```python
from build123d import *

# Parameters (mm, degrees)
SKETCH1_W           = 37.9349
SKETCH1_H           = 37.9349
BOSS_EXTRUDE1_DEPTH = 3.175
SKETCH9_R           = 1.1176
CUT_EXTRUDE2_DEPTH  = 3.175
SKETCH10_R          = 7.493
CUT_EXTRUDE3_DEPTH  = 3.175
SKETCH11_W          = 10.4648
SKETCH11_H          = 1.8796
BOSS_EXTRUDE2_DEPTH = 3.175


with BuildPart() as part:
    # Sketch1 → Boss-Extrude1 (new body)
    with BuildSketch(Plane.XY):
        with Locations((18.96745, 18.96745)):
            Rectangle(SKETCH1_W, SKETCH1_H)
    extrude(amount=BOSS_EXTRUDE1_DEPTH)

    # Sketch9 → Cut-Extrude2 (cut)
    with BuildSketch(Plane.XY.offset(3.175)):
        with Locations((33.62325, 33.62325)):
            Circle(SKETCH9_R)
        with Locations((4.31165, 33.62325)):
            Circle(SKETCH9_R)
        with Locations((4.31165, 4.31165)):
            Circle(SKETCH9_R)
        with Locations((33.62325, 4.31165)):
            Circle(SKETCH9_R)
        with BuildLine():
            Line((35.385619933, 12.100169933), (35.385619933, 2.549280067))
            Line((35.385619933, 2.549280067), (25.834730067, 2.549280067))
            ThreePointArc((25.834730067, 2.549280067), (25.2984, 2.01295), (25.834730067, 1.476619933))
            Line((25.834730067, 1.476619933), (35.385619933, 1.476619933))
            ThreePointArc((35.385619933, 1.476619933), (37.303202335, 0.631697665), (36.458280067, 2.549280067))
            Line((36.458280067, 2.549280067), (36.458280067, 12.100169933))
            ThreePointArc((36.458280067, 12.100169933), (35.92195, 12.6365), (35.385619933, 12.100169933))
        make_face()
        with BuildLine():
            Line((35.385619933, 36.458280067), (25.834730067, 36.458280067))
            ThreePointArc((25.834730067, 36.458280067), (25.2984, 35.92195), (25.834730067, 35.385619933))
            Line((25.834730067, 35.385619933), (35.385619933, 35.385619933))
            Line((35.385619933, 35.385619933), (35.385619933, 25.834730067))
            ThreePointArc((35.385619933, 25.834730067), (35.92195, 25.2984), (36.458280067, 25.834730067))
            Line((36.458280067, 25.834730067), (36.458280067, 35.385619933))
            ThreePointArc((36.458280067, 35.385619933), (37.303202335, 37.303202335), (35.385619933, 36.458280067))
        make_face()
        with BuildLine():
            Line((12.048880067, 36.458280067), (2.549280067, 36.458280067))
            ThreePointArc((2.549280067, 36.458280067), (0.631697665, 37.303202335), (1.476619933, 35.385619933))
            Line((1.476619933, 35.385619933), (1.476619933, 25.886019933))
            ThreePointArc((1.476619933, 25.886019933), (2.01295, 25.349689867), (2.549280067, 25.886019933))
            Line((2.549280067, 25.886019933), (2.549280067, 35.385619933))
            Line((2.549280067, 35.385619933), (12.048880067, 35.385619933))
            ThreePointArc((12.048880067, 35.385619933), (12.585210133, 35.92195), (12.048880067, 36.458280067))
        make_face()
        with BuildLine():
            Line((23.06955, 36.458280067), (14.86535, 36.458280067))
            ThreePointArc((14.86535, 36.458280067), (14.329019933, 35.92195), (14.86535, 35.385619933))
            Line((14.86535, 35.385619933), (23.06955, 35.385619933))
            ThreePointArc((23.06955, 35.385619933), (23.605880067, 35.92195), (23.06955, 36.458280067))
        make_face()
        with BuildLine():
            Line((2.549280067, 23.06955), (2.549280067, 14.86535))
            ThreePointArc((2.549280067, 14.86535), (2.01295, 14.329019933), (1.476619933, 14.86535))
            Line((1.476619933, 14.86535), (1.476619933, 23.06955))
            ThreePointArc((1.476619933, 23.06955), (2.01295, 23.605880067), (2.549280067, 23.06955))
        make_face()
        with BuildLine():
            Line((36.458280067, 23.06955), (36.458280067, 14.86535))
            ThreePointArc((36.458280067, 14.86535), (35.92195, 14.329019933), (35.385619933, 14.86535))
            Line((35.385619933, 14.86535), (35.385619933, 23.06955))
            ThreePointArc((35.385619933, 23.06955), (35.92195, 23.605880067), (36.458280067, 23.06955))
        make_face()
        with BuildLine():
            Line((23.06955, 2.549280067), (14.86535, 2.549280067))
            ThreePointArc((14.86535, 2.549280067), (14.329019933, 2.01295), (14.86535, 1.476619933))
            Line((14.86535, 1.476619933), (23.06955, 1.476619933))
            ThreePointArc((23.06955, 1.476619933), (23.605880067, 2.01295), (23.06955, 2.549280067))
        make_face()
        with BuildLine():
            Line((2.549280067, 12.100169933), (2.549280067, 2.549280067))
            Line((2.549280067, 2.549280067), (12.100169933, 2.549280067))
            ThreePointArc((12.100169933, 2.549280067), (12.6365, 2.01295), (12.100169933, 1.476619933))
            Line((12.100169933, 1.476619933), (2.600569933, 1.476619933))
            ThreePointArc((2.600569933, 1.476619933), (0.681867267, 0.681867267), (1.476619933, 2.600569933))
            Line((1.476619933, 2.600569933), (1.476619933, 12.100169933))
            ThreePointArc((1.476619933, 12.100169933), (2.01295, 12.6365), (2.549280067, 12.100169933))
        make_face()
    extrude(amount=-CUT_EXTRUDE2_DEPTH, mode=Mode.SUBTRACT)

    # Sketch10 → Cut-Extrude3 (cut)
    with BuildSketch(Plane(origin=(0, 0, 0), x_dir=(-1, 0, 0), z_dir=(0, 0, -1))):
        with Locations((-18.96745, 18.96745)):
            Circle(SKETCH10_R)
    extrude(amount=-CUT_EXTRUDE3_DEPTH, mode=Mode.SUBTRACT)

    # Sketch11 → Boss-Extrude2 (add)
    with BuildSketch(Plane.XY.offset(3.175)):
        with Locations((-5.2324, 25.8191)):
            Rectangle(SKETCH11_W, SKETCH11_H)
        with Locations((-5.2324, 12.1158)):
            Rectangle(SKETCH11_W, SKETCH11_H)
    extrude(amount=-BOSS_EXTRUDE2_DEPTH)


solid = part.part
```
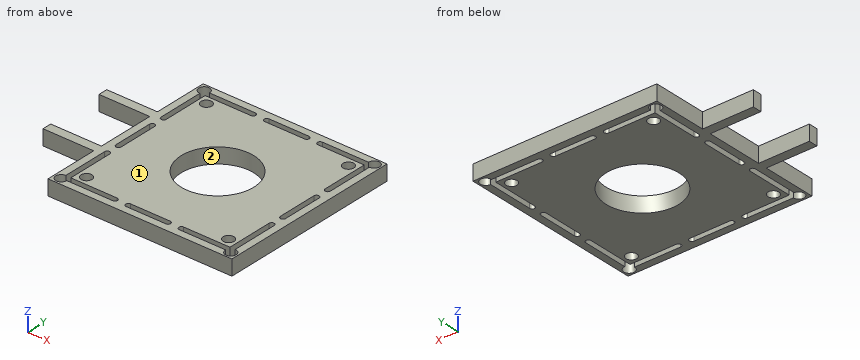
Could you check a few things on this model? Use its own coordinates, in mm. Face numbers are marked on the shaded views. Round coordinates to 2 decimals unless told otherwise and drop trailing zeros. Loops run counter-clockwise (first coordinate to the right, second up) from the corner with the lowest first, then second, coordinate; pieces in that order, holes last. Notation, with made-up numbers: M 80.25,-30 L 115.25,-30 A25 ccw 115.25,2 Z; hole C -10.75,11.5 d10. An arc over 180 degrees is marked long. Put each result on its own line as item: value.
Q1. Imagine slicing it at D-D (x = 22.5). Write out the boundary of the cut face in (y, z) (3 decimals).
Check result:
outline: M 0,0 L 1.477,0 L 1.477,3.175 L 0,3.175 Z; M 2.549,0 L 12.359,0 L 12.359,3.175 L 2.549,3.175 Z; M 25.575,0 L 35.386,0 L 35.386,3.175 L 25.575,3.175 Z; M 36.458,0 L 37.935,0 L 37.935,3.175 L 36.458,3.175 Z
Q2. Thinking about a two-plate mould opening in Y: for the marked faces 1 and 2, which applies, released by +Y, released by -Y, zero draft, split by the parting line, or undercut?
Check result:
face 1: zero draft
face 2: undercut
Q3. I need wall thicknesses on probe 1 along X at (y, z) = (35, 0.9); probe 2 along X at (y, z) = (19, 0.6). Which ranges of each line are inside material? Lowest first, please.
Check result:
probe 1: 0 to 1.48, 2.55 to 35.39, 36.46 to 37.93
probe 2: 0 to 1.48, 2.55 to 11.47, 26.46 to 35.39, 36.46 to 37.93
Q4. For pin 1 (1 mm diameter, centred on y = 7.5, z = 2, fed in from -X); pin 2 (2 mm diameter, centred on x = 36.51, y = 1.43, fed in from -Z); pin 3 (1 mm diameter, centred on x = -4, z = 1, fed in from -Y), each with a flat end and sliding along its axis, tell me the tip position at first contact or that it passes through.
Check result:
pin 1: x = 0
pin 2: through
pin 3: y = 11.18
Q5. Imagine slicing it at C-C (y = 16). Write out the boundary of the cut face in (x, z) (3 decimals), then the cut area to 3 significant figures.
Check result:
outline: M 0,0 L 1.477,0 L 1.477,3.175 L 0,3.175 Z; M 2.549,0 L 12.087,0 L 12.087,3.175 L 2.549,3.175 Z; M 25.848,0 L 35.386,0 L 35.386,3.175 L 25.848,3.175 Z; M 36.458,0 L 37.935,0 L 37.935,3.175 L 36.458,3.175 Z
area: 69.9 mm2
Q6. Imagine slicing it at A-A (x = 27.5). Write out the boundary of the cut face in (y, z) (3 decimals).
Check result:
outline: M 0,0 L 1.477,0 L 1.477,3.175 L 0,3.175 Z; M 2.549,0 L 35.386,0 L 35.386,3.175 L 2.549,3.175 Z; M 36.458,0 L 37.935,0 L 37.935,3.175 L 36.458,3.175 Z
